Source: CAD feature listing. Evaluate the final solid. Frame: model axes, mm. Face numbers are marked on the shaded views. A direction names the side the tool comes from. Coordinates: 2 decimals unless noted, no trailing zeros. Write each loop counter-clockwise with the first axis right and the second up, starting at its lowest first coordinate (ties: lowest second). Pieces come first, ordered by that corner, then holes. Notation, with made-up numbers: (5.25, -38) - (30.25, -38) arc R19 ccw to (30.25, -23) - close; hole circle Ø7 at (7.5, -18.75). An arc over 180 degrees is marked (long way). One line per question, with ' | ' between items.
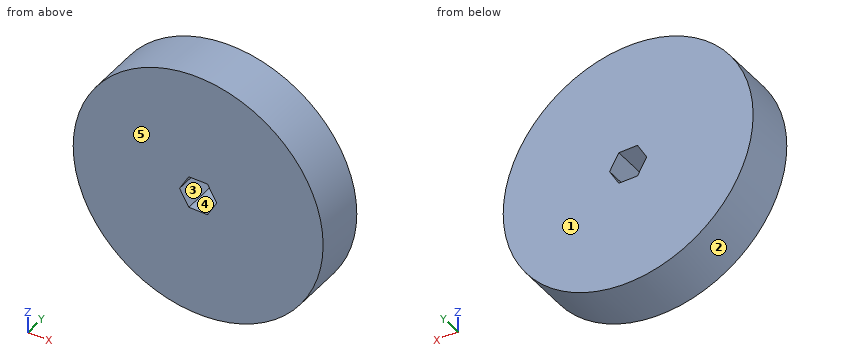
Solid Edge part; units mm, degrees
sketch "Sketch1" plane through (0, 0, 0) normal (0, -1, 0) x (1, 0, 0)
  circle A0 centre (0, 0) radius 49.2125
extrude "Protrusion1" add sketch "Sketch1" along normal blind 20.32
sketch "Sketch2" plane through (0, -20.32, 0) normal (0, -1, 0) x (1, 0, 0)
  line L0 (-3.6639, 6.3461) -> (3.6639, 6.3461)
  line L1 (3.6639, 6.3461) -> (7.3279, 0)
  line L2 (7.3279, 0) -> (3.664, -6.3461)
  line L3 (3.664, -6.3461) -> (-3.6639, -6.3461)
  line L4 (-3.6639, -6.3461) -> (-7.3279, 0)
  line L5 (-7.3279, 0) -> (-3.6639, 6.3461)
extrude "Cutout1" cut sketch "Sketch2" against normal up to next
Item 1: Pin query (flat end, axial travel): pin 1 Ø12 at (x, y) = (4, -13.5) entering from -Z; pin 2 Ø12 at (y, z) = (-8.5, -16) entering from +X; pin 3 Ø2 at (x, y) = (-0.5, -5.5) entering from +Z; pin 4 Ø5 at (y, z) = (-9.5, -2) entering from -X. Return the tip coordinate at first contact, or that it passes through.
Check sheet entries:
pin 1: z = -49.21 | pin 2: x = 48.19 | pin 3: z = 49.21 | pin 4: x = -49.21
Item 2: Ray query, line 1 along X through (y, z) = (-11.5, -3.5); line 2 along X through (y, z) = (-7.5, -5); line 3 along X through (y, z) = (-11, 7.5). Return the intervals inside material, ascending. Write a range as [from, to].
Check sheet entries:
line 1: [-49.09, -5.31], [5.31, 49.09] | line 2: [-48.96, -4.44], [4.44, 48.96] | line 3: [-48.64, 48.64]
Item 3: Cut plane D-D on x = -17. Return loops of the section in (y, z).
Check sheet entries:
outline: (-20.32, -46.18) - (0, -46.18) - (0, 46.18) - (-20.32, 46.18) - close
Item 4: Cut plane C-C on z = -29. Return loops of the section in (x, y).
Check sheet entries:
outline: (-39.76, -20.32) - (39.76, -20.32) - (39.76, 0) - (-39.76, 0) - close
Item 5: Cut plane A-A on x = 0. Return loops of the section in (y, z).
Check sheet entries:
outline: (-20.32, -49.21) - (0, -49.21) - (0, -6.35) - (-20.32, -6.35) - close; (-20.32, 6.35) - (0, 6.35) - (0, 49.21) - (-20.32, 49.21) - close
Item 6: Cut plane B-B on y = -4.5. Return loops of the section in (x, z) (1 decimal).
Check sheet entries:
outline: circle Ø98.4 at (0, 0); hole (-7.3, 0) - (-3.7, -6.3) - (3.7, -6.3) - (7.3, 0) - (3.7, 6.3) - (-3.7, 6.3) - close
Item 7: Mould query, pull axis Z, two halves, no side actions, for the marked faces 1, 2 and 3. Classes: pulls with the +Z half, pulls with the -Z half, needs draft (parallel to the pull), parting line crosses it, or undercut.
Check sheet entries:
face 1: needs draft | face 2: parting line crosses it | face 3: undercut
Item 8: Access query for the marked faces 4 and 5. Directions: +Z, -Z, +X, -X, +Y, -Y. A direction counts if a zero-diameter tool reaches every point of the face in a straight line with its end or side. Return the directions, or none.
Check sheet entries:
face 4: +Y, -Y | face 5: +Z, -Z, +X, -X, -Y
